Autodesk Inventor part; units mm, degrees
ref_plane "YZ Plane" through (0, 0, 0) normal (1, 0, 0) x (0, 1, 0)
ref_plane "XZ Plane" through (0, 0, 0) normal (0, 1, 0) x (-1, 0, 0)
ref_plane "XY Plane" through (0, 0, 0) normal (0, 0, 1) x (1, 0, 0)
sketch "Sketch1" plane through (0, 0, 0) normal (0, 1, 0) x (-1, 0, 0)
  line L0 (-50, -50) -> (50, -50)
  line L1 (50, -50) -> (50, 50)
  line L2 (50, 50) -> (-50, 50)
  line L3 (-50, 50) -> (-50, -50)
  line L4 (-50, -50) -> (50, 50) construction
  line L5 (50, -50) -> (-50, 50) construction
  point P0 (0, 0)
  dimension "d2" = 100
  dimension "d3" = 100
extrude "Extrusion1" add sketch "Sketch1" along normal blind 5
sketch "Sketch2" plane through (0, 5, 0) normal (0, 1, 0) x (1, 0, 0)
  line L0 (-50, 50) -> (-50, -50)
  line L1 (-50, -50) -> (50, -50)
  line L2 (50, -50) -> (50, 50)
  line L3 (50, 50) -> (-50, 50)
  line L4 (47, 47) -> (-47, 47)
  line L5 (-47, 47) -> (-47, -47)
  line L6 (-47, -47) -> (47, -47)
  line L7 (47, -47) -> (47, 47)
  line L8 (47, 47) -> (-47, -47) construction
  line L9 (-47, 47) -> (47, -47) construction
  line L10 (45, 45) -> (-45, 45)
  line L11 (-45, 45) -> (-45, -45)
  line L12 (-45, -45) -> (45, -45)
  line L13 (45, -45) -> (45, 45)
  line L14 (45, 45) -> (-45, -45) construction
  line L15 (-45, 45) -> (45, -45) construction
  point P0 (0, 0)
  dimension "d6" = 3
  dimension "d7" = 2
extrude "Extrusion2" add sketch "Sketch2" along normal blind 40 contours L7 L6 L5 L4
fillet "Fillet1" radius 1 1 edges at (50, 2.5, 50)
fillet "Fillet2" radius 1 1 edges at (50, 2.5, -50)
fillet "Fillet3" radius 1 1 edges at (-50, 2.5, 50)
fillet "Fillet4" radius 1 1 edges at (-50, 2.5, -50)
fillet "Fillet5" radius 1 1 edges at (-47, 25, 47)
fillet "Fillet6" radius 1 1 edges at (47, 25, 47)
fillet "Fillet7" radius 1 1 edges at (47, 25, -47)
fillet "Fillet8" radius 1 1 edges at (-47, 25, -47)
sketch "Sketch3" plane through (0, 45, 0) normal (0, 1, 0) x (1, 0, 0)
  arc A0 (-46, 47) -> (-47, 46) centre (-46, 46) ccw
  line L0 (-47, 46) -> (-47, -46)
  arc A1 (-47, -46) -> (-46, -47) centre (-46, -46) ccw
  line L1 (-46, -47) -> (46, -47)
  arc A2 (46, -47) -> (47, -46) centre (46, -46) ccw
  line L2 (47, -46) -> (47, 46)
  arc A3 (47, 46) -> (46, 47) centre (46, 46) ccw
  line L3 (46, 47) -> (-46, 47)
  line L4 (45, 45) -> (45, -45)
  line L5 (45, -45) -> (-45, -45)
  line L6 (-45, -45) -> (-45, 45)
  line L7 (-45, 45) -> (45, 45)
  line L8 (-46.5, -40) -> (-45.5, -40)
  line L9 (-45.5, -40) -> (-45.5, -20)
  line L10 (-45.5, -20) -> (-46.5, -20)
  line L11 (-46.5, -20) -> (-46.5, -40)
  line L12 (-46.5, 40) -> (-45.5, 40)
  line L13 (-45.5, 40) -> (-45.5, 20)
  line L14 (-45.5, 20) -> (-46.5, 20)
  line L15 (-46.5, 20) -> (-46.5, 40)
  line L16 (-40, 46.5) -> (-20, 46.5)
  line L17 (-20, 46.5) -> (-20, 45.5)
  line L18 (-20, 45.5) -> (-40, 45.5)
  line L19 (-40, 45.5) -> (-40, 46.5)
  line L20 (40, 46.5) -> (20, 46.5)
  line L21 (20, 46.5) -> (20, 45.5)
  line L22 (20, 45.5) -> (40, 45.5)
  line L23 (40, 45.5) -> (40, 46.5)
  line L24 (45.5, 40) -> (46.5, 40)
  line L25 (46.5, 40) -> (46.5, 20)
  line L26 (46.5, 20) -> (45.5, 20)
  line L27 (45.5, 20) -> (45.5, 40)
  line L28 (45.5, -40) -> (46.5, -40)
  line L29 (46.5, -40) -> (46.5, -20)
  line L30 (46.5, -20) -> (45.5, -20)
  line L31 (45.5, -20) -> (45.5, -40)
  line L32 (40, -45.5) -> (20, -45.5)
  line L33 (20, -45.5) -> (20, -46.5)
  line L34 (20, -46.5) -> (40, -46.5)
  line L35 (40, -46.5) -> (40, -45.5)
  line L36 (-40, -45.5) -> (-20, -45.5)
  line L37 (-20, -45.5) -> (-20, -46.5)
  line L38 (-20, -46.5) -> (-40, -46.5)
  line L39 (-40, -46.5) -> (-40, -45.5)
  point P0 (0, 0)
  point P1 (-46, 40)
  point P2 (-46, 20)
  point P3 (46, 40)
  dimension "d18" = 1
  dimension "d19" = 20
  dimension "d20" = 0.5
  dimension "d21" = 7
  dimension "d22" = 7
  dimension "d23" = 0.5
  dimension "d24" = 1
  dimension "d25" = 20
  dimension "d26" = 20
  dimension "d27" = 1
  dimension "d28" = 0.5
  dimension "d29" = 7
  dimension "d30" = 20
  dimension "d31" = 1
  dimension "d32" = 0.5
  dimension "d33" = 7
  dimension "d34" = 1
  dimension "d35" = 20
  dimension "d36" = 0.5
  dimension "d37" = 7
  dimension "d38" = 1
  dimension "d39" = 20
  dimension "d40" = 7
  dimension "d41" = 0.5
  dimension "d42" = 20
  dimension "d43" = 1
  dimension "d44" = 0.5
  dimension "d45" = 7
  dimension "d46" = 20
  dimension "d47" = 1
  dimension "d48" = 0.5
  dimension "d49" = 7
extrude "Extrusion3" cut sketch "Sketch3" against normal blind 1 contours L11 L10 L9 L8 | L12 L13 L14 L15 | L16 L17 L18 L19 | L23 L22 L21 L20 | L24 L25 L26 L27 | L31 L30 L29 L28 | L35 L34 L33 L32 | L36 L37 L38 L39
properties part number "block_main" material "PC/ABS Plastic"
Design review of the part built by this model. Coordinates are the model's own, in mm. A direction names the side the tool comes from. Coordinates: 2 decimals unless noted, no trailing zeros. Order: outer loops, then holes, each group sorted by start corner. A loop starts at its lowest first (then second) coordinate and runs counter-clockwise, first axis right, second up.
1) Wall thickness on line 1 along Z through (x, y) = (23, 36); line 2 along Y through (x, z) = (8.5, 26): over which ranges is each line inside the solid? List them lowest first.
2) Take a section at C-C, the plane z = -27. Give the boundary of the cut face in (x, y).
3) Take a section at A-A, the plane y = 8.5. Give the boundary of the cut face in (x, z).
4) Clearance check with flat-ended pins moving along their axes: pin 1 (8 mm diameter, centred on y = 17, z = 11, fed in from -X); pin 2 (6 mm diameter, centred on x = 11.5, z = -0.5, fed in from +Y); pin 3 (0.5 mm diameter, centred on x = 46, y = 44.5, fed in from +Z). State where each tip first meets the part, or that it passes through.
5) Mouldability with a two-part tool opening along X and no side actions: class faces 1 (the flat face through (47, 25, 1)), 2 (the flat face through (45, 25, 1)), 3 (the flat face through (1, 0, 1)) as +X half, -X half, draft (parallel to the pull), parting line (faces both ways), or undercut.
6) Take a section at B-B, the plane x = -15.5. Give the boundary of the cut face in (y, z), and give its area (3 significant figures).
7) For faces 4 (the flat face through (-1, 25, 45)), 5 (the flat face through (1, 25, -47)), 6 (the flat face through (-47, 25, -1)), 7 (the flat face through (-1, 25, 47)), list the 3-axis set-ups (+Z, -Z, +X, -X, +Y, -Y) from which the entire face can be reached by the end or side of a thin tool; tool diameter is ignored.
8) Take a section at D-D, the plane z = 9.5. Give the boundary of the cut face in (x, y).
Returned:
1. line 1: z = -47 to -45, 45 to 47
1. line 2: y = 0 to 5
2. outline: (-50, 0) - (50, 0) - (50, 5) - (47, 5) - (47, 45) - (46.5, 45) - (46.5, 44) - (45.5, 44) - (45.5, 45) - (45, 45) - (45, 5) - (-45, 5) - (-45, 45) - (-45.5, 45) - (-45.5, 44) - (-46.5, 44) - (-46.5, 45) - (-47, 45) - (-47, 5) - (-50, 5) - close
3. outline: (-47, -46) arc R1 ccw to (-46, -47) - (46, -47) arc R1 ccw to (47, -46) - (47, 46) arc R1 ccw to (46, 47) - (-46, 47) arc R1 ccw to (-47, 46) - close; hole (-45, -45) - (45, -45) - (45, 45) - (-45, 45) - close
4. pin 1: stops at x = -47
4. pin 2: stops at y = 5
4. pin 3: stops at z = 47
5. face 1: +X half
5. face 2: undercut
5. face 3: draft
6. outline: (0, -50) - (5, -50) - (5, -47) - (45, -47) - (45, -45) - (5, -45) - (5, 45) - (45, 45) - (45, 47) - (5, 47) - (5, 50) - (0, 50) - close
6. area: 660 mm2
7. face 4: +Y
7. face 5: -Z, +X, -X, +Y
7. face 6: +Z, -Z, -X, +Y
7. face 7: +Z, +X, -X, +Y
8. outline: (-50, 0) - (50, 0) - (50, 5) - (47, 5) - (47, 45) - (45, 45) - (45, 5) - (-45, 5) - (-45, 45) - (-47, 45) - (-47, 5) - (-50, 5) - close
